from build123d import *

# Parameters (mm, degrees)
SKETCH_2_R               = 2.3
CUT_EXTRUDE_1_DEPTH      = 10
PATTERN_CIRCULAR_1_COUNT = 8


with BuildPart() as part:
    # 草图1 → 旋转1 (revolve)
    with BuildSketch(Plane.XY):
        Polygon((-93.5, 3.4), (-93.5, 0), (-73.1, 0), (-71.429545455, 21), (-74, 21), (-75.4, 3.4), align=None)
        with BuildLine():
            ThreePointArc((0, 92.429545455), (-50.508315968, 71.508315968), (-71.429545455, 21))
            Line((-71.429545455, 21), (-74, 21))
            ThreePointArc((-74, 21), (-52.325901808, 73.325901808), (0, 95))
            Line((0, 95), (0, 92.429545455))
        make_face()
        Polygon((-79.5, 4.4), (-80.077350269, 3.4), (-78.922649731, 3.4), align=None)
    revolve(axis=Axis((0, 0, 0), (0, 1, 0)))

    # 草图2 → 切除-拉伸1 (cut)
    with BuildSketch(Plane(origin=(0, 3.4, 0), x_dir=(1, 0, 0), z_dir=(0, 1, 0))):
        with Locations((0, 86)):
            Circle(SKETCH_2_R)
    cut_extrude_1 = extrude(amount=-CUT_EXTRUDE_1_DEPTH, mode=Mode.SUBTRACT)

    # 阵列(圆周)1: 切除-拉伸1 ×8 about axis
    pattern_circular_1_axis = Axis((0, 0, 0), (0, 1, 0))
    for i in range(1, PATTERN_CIRCULAR_1_COUNT):
        add(cut_extrude_1.rotate(pattern_circular_1_axis, i * 360 / PATTERN_CIRCULAR_1_COUNT), mode=Mode.SUBTRACT)


solid = part.part
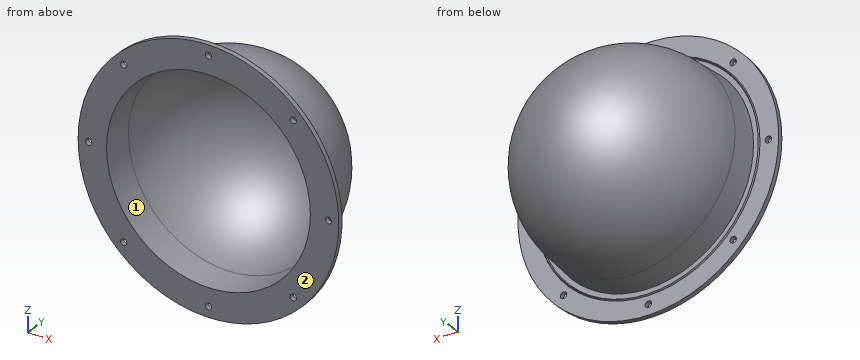
Work out the finished part from the listing and answer in its coordinate system (mm). Face numbers are marked on the shaded views. Coordinates: 2 decimals unless noted, no trailing zeros. Write each loop counter-clockwise with the first axis right and the second up, starting at its lowest first coordinate (ties: lowest second). Pieces come first, ordered by that corner, then holes.
1. The part is cut by section A-A, the plane x = 0. Write down the section's boundary in (y, z).
Results list:
outline: (0, -93.5) - (3.4, -93.5) - (3.4, -88.3) - (0, -88.3) - close; (0, -83.7) - (3.4, -83.7) - (3.4, -80.08) - (4.4, -79.5) - (3.4, -78.92) - (3.4, -75.4) - (21, -74) arc R74 ccw to (21, 74) - (3.4, 75.4) - (3.4, 78.92) - (4.4, 79.5) - (3.4, 80.08) - (3.4, 83.7) - (0, 83.7) - (0, 73.1) - (21, 71.43) arc R71.43 cw to (21, -71.43) - (0, -73.1) - close; (0, 88.3) - (3.4, 88.3) - (3.4, 93.5) - (0, 93.5) - close
2. The part is cut by section D-D, the plane z = 86. Write down the section's boundary in (x, y), and give its area (3 significant figures).
Results list:
outline: (-36.69, 0) - (-2.3, 0) - (-2.3, 3.4) - (-36.69, 3.4) - close; (2.3, 0) - (36.69, 0) - (36.69, 3.4) - (2.3, 3.4) - close
area: 234 mm2
3. The part is cut by section B-B, the plane z = 0. Write down the section's boundary in (x, y).
Results list:
outline: (-93.5, 0) - (-88.3, 0) - (-88.3, 3.4) - (-93.5, 3.4) - close; (-83.7, 0) - (-73.1, 0) - (-71.43, 21) arc R71.43 cw to (71.43, 21) - (73.1, 0) - (83.7, 0) - (83.7, 3.4) - (80.08, 3.4) - (79.5, 4.4) - (78.92, 3.4) - (75.4, 3.4) - (74, 21) arc R74 ccw to (-74, 21) - (-75.4, 3.4) - (-78.92, 3.4) - (-79.5, 4.4) - (-80.08, 3.4) - (-83.7, 3.4) - close; (88.3, 0) - (93.5, 0) - (93.5, 3.4) - (88.3, 3.4) - close
4. Flat-ended cylindrical pins translate along their axes: pin 1 (7.5 mm diameter, centred on x = 0, z = -86, fed in from +Y); pin 2 (12 mm diameter, centred on x = -11, z = -10.5, fed in from -Y); pin 3 (3.5 mm diameter, centred on x = 60.81, z = 60.81, fed in from +Y); pin 4 (1 mm diameter, centred on y = 18, z = 63, fed in from +X). Find the tip coordinate at first contact, or state that the pin passes through.
Results list:
pin 1: stops at y = 3.4
pin 2: stops at y = 89.21
pin 3: passes through
pin 4: stops at x = 40.07
5. Consider line 1 along Z through (x, y) = (0, 2.65); line 2 along X through (y, z) = (15.5, -52); line 3 along X through (y, z) = (24.5, -54). Determine where each line is inside the solid, lowest interval first.
Results list:
line 1: z = -93.5 to -88.3, -83.7 to -72.89, 72.89 to 83.7, 88.3 to 93.5
line 2: x = -53.26 to -49.61, 49.61 to 53.26
line 3: x = -50.48 to -46.63, 46.63 to 50.48
6. For a pull along Z with two mould halves and no side action, classify the marked faces 1 and 2 as +Z half, -Z half, draft (parallel to the pull), parting line (faces both ways), or undercut.
Results list:
face 1: undercut
face 2: draft
7. The part is cut by section C-C, the plane x = 86. Write down the section's boundary in (y, z), and give its area (3 significant figures).
Results list:
outline: (0, -36.69) - (3.4, -36.69) - (3.4, -2.3) - (0, -2.3) - close; (0, 2.3) - (3.4, 2.3) - (3.4, 36.69) - (0, 36.69) - close
area: 234 mm2
